from build123d import *

# Parameters (mm, degrees)
SKETCH1_W           = 48.698269881
SKETCH1_H           = 79.9
SKETCH1_W_2         = 13.312275424
SKETCH1_H_2         = 6.8
SKETCH1_W_3         = 7
SKETCH1_H_3         = 6.6
SKETCH1_W_4         = 10.999995004
SKETCH1_H_4         = 49.999979698
BOSS_EXTRUDE1_DEPTH = 6


with BuildPart() as part:
    # Sketch1 → Boss-Extrude1 (new body)
    with BuildSketch(Plane.XY):
        with Locations((-328.119749272, -326.315940756)):
            Rectangle(SKETCH1_W, SKETCH1_H)
        Polygon((-306.547681314, -310.331815037), (-306.727502074, -310.765940756), (-307.013555595, -311.138732962), (-307.386347801, -311.424786483), (-307.82047352, -311.604607243), (-308.286347801, -311.665940756), (-308.752222082, -311.604607243), (-309.186347801, -311.424786483), (-309.559140007, -311.138732962), (-309.845193528, -310.765940756), (-310.025014288, -310.331815037), (-310.086347801, -309.865940756), (-310.025014288, -309.400066475), (-309.845193528, -308.965940756), (-309.559140007, -308.59314855), (-309.186347801, -308.307095029), (-308.752222082, -308.127274269), (-308.286347801, -308.065940756), (-307.82047352, -308.127274269), (-307.386347801, -308.307095029), (-307.013555595, -308.59314855), (-306.727502074, -308.965940756), (-306.547681314, -309.400066475), (-306.486347801, -309.865940756), align=None, mode=Mode.SUBTRACT)
        with Locations((-314.125021924, -356.265940756)):
            Rectangle(SKETCH1_W_2, SKETCH1_H_2, mode=Mode.SUBTRACT)
        with Locations((-344.168884212, -356.165940756)):
            Rectangle(SKETCH1_W_3, SKETCH1_H_3, mode=Mode.SUBTRACT)
        with Locations((-314.125021924, -296.365940756)):
            Rectangle(SKETCH1_W_2, SKETCH1_H_2, mode=Mode.SUBTRACT)
        Polygon((-349.005509995, -349.753374061), (-349.195776334, -349.323723778), (-349.268357829, -348.859468921), (-349.218308171, -348.392247692), (-349.04903816, -347.953900444), (-348.77208327, -347.574299819), (-348.406317517, -347.279314973), (-347.976667234, -347.089048634), (-347.512412377, -347.016467139), (-347.045191148, -347.066516797), (-346.6068439, -347.235786808), (-346.227243275, -347.512741698), (-345.932258429, -347.878507451), (-345.74199209, -348.308157734), (-345.669410595, -348.772412591), (-345.719460253, -349.23963382), (-345.888730263, -349.677981068), (-346.165685154, -350.057581692), (-346.531450907, -350.352566539), (-346.96110119, -350.542832878), (-347.425356047, -350.615414373), (-347.892577276, -350.565364715), (-348.330924524, -350.396094704), (-348.710525148, -350.119139814), align=None, mode=Mode.SUBTRACT)
        Polygon((-307.013555595, -341.49314855), (-306.727502074, -341.865940756), (-306.547681314, -342.300066475), (-306.486347801, -342.765940756), (-306.547681314, -343.231815037), (-306.727502074, -343.665940756), (-307.013555595, -344.038732962), (-307.386347801, -344.324786483), (-307.82047352, -344.504607243), (-308.286347801, -344.565940756), (-308.752222082, -344.504607243), (-309.186347801, -344.324786483), (-309.559140007, -344.038732962), (-309.845193528, -343.665940756), (-310.025014288, -343.231815037), (-310.086347801, -342.765940756), (-310.025014288, -342.300066475), (-309.845193528, -341.865940756), (-309.559140007, -341.49314855), (-309.186347801, -341.207095029), (-308.752222082, -341.027274269), (-308.286347801, -340.965940756), (-307.82047352, -341.027274269), (-307.386347801, -341.207095029), align=None, mode=Mode.SUBTRACT)
        Polygon((-347.042471777, -302.06717764), (-346.604388229, -302.237128957), (-346.225218653, -302.51467369), (-345.93080283, -302.880897622), (-345.741204711, -303.310843199), (-345.669345095, -303.77521034), (-345.720121096, -304.242353191), (-345.890072413, -304.680436739), (-346.167617146, -305.059606315), (-346.533841078, -305.354022138), (-346.963786655, -305.543620257), (-347.428153795, -305.615479873), (-347.895296647, -305.564703872), (-348.333380195, -305.394752555), (-348.712549771, -305.117207822), (-349.006965594, -304.75098389), (-349.196563713, -304.321038313), (-349.268423329, -303.856671172), (-349.217647328, -303.389528321), (-349.047696011, -302.951444773), (-348.770151278, -302.572275197), (-348.403927346, -302.277859374), (-347.973981769, -302.088261255), (-347.509614628, -302.016401639), align=None, mode=Mode.SUBTRACT)
        with Locations((-344.168884212, -296.365940756)):
            Rectangle(SKETCH1_W_3, SKETCH1_H_2, mode=Mode.SUBTRACT)
        with Locations((-330.086347801, -326.315940756)):
            Rectangle(SKETCH1_W_4, SKETCH1_H_4, mode=Mode.SUBTRACT)
    extrude(amount=BOSS_EXTRUDE1_DEPTH)


solid = part.part
Could you check a few things on this model? Use its own coordinates, in mm. A direction names the side the tool comes from. Coordinates: 2 decimals unless noted, no trailing zeros. Loops run counter-clockwise (first coordinate to the right, second up) from the corner with the lowest first, then second, coordinate; pieces in that order, holes last.
1. Imagine slicing it at C-C (x = -333). Please give me the cut outline in (y, z), and give its area (3 significant figures).
2. I need wall thicknesses on L1, parallel to Y at x = -343, z = 1.8; L2, parallel to Y at x = -312.5, z = 0.6; L3, parallel to X at y = -332, z = 2.05. Which ranges of each line are inside material? Lowest first, please.
3. Imagine slicing it at D-D (z = 3.15). Give the number of separate pieces and of enclosed holes in the cut face, and give its area (3 significant figures).
4. Imagine slicing it at B-B (y = -330.5). Please give me the cut outline in (x, z).
5. Imagine slicing it at A-A (x = -314.5). Please give me the cut outline in (y, z).
6. For faces 3 (the face through (-344, -352.866, 3)), 4 (the face through (-323, -326, 6)), which set-ups out of +Z, -Z, +X, -X, +Y, -Y let a thin tool reach every point of the face, with its end or its side?
7. For P1, Ø6, axis at x = -337.5, y = -299, coming from the -Z side, with a flat end and sliding along its axis, tell me the tip position at first contact or that it passes through.
8. We'd pull the mould along Y, two halves only. Please class faces 1 (the face through (-335.586, -327, 3)), 2 (the face through (-323, -326, 0)): released by +Y, released by -Y, zero draft, split by the parting line, or undercut.
Computed values:
1. outline: (-366.27, 0) - (-351.32, 0) - (-351.32, 6) - (-366.27, 6) - close; (-301.32, 0) - (-286.37, 0) - (-286.37, 6) - (-301.32, 6) - close
1. area: 179 mm2
2. L1: y = -366.27 to -359.47, -352.87 to -299.77, -292.97 to -286.37
2. L2: y = -366.27 to -359.67, -352.87 to -299.77, -292.97 to -286.37
2. L3: x = -352.47 to -335.59, -324.59 to -303.77
3. separate pieces: 1
3. enclosed holes: 9
3. area: 3,030 mm2
4. outline: (-352.47, 0) - (-335.59, 0) - (-335.59, 6) - (-352.47, 6) - close; (-324.59, 0) - (-303.77, 0) - (-303.77, 6) - (-324.59, 6) - close
5. outline: (-366.27, 0) - (-359.67, 0) - (-359.67, 6) - (-366.27, 6) - close; (-352.87, 0) - (-299.77, 0) - (-299.77, 6) - (-352.87, 6) - close; (-292.97, 0) - (-286.37, 0) - (-286.37, 6) - (-292.97, 6) - close
6. face 3: +Z, -Z
6. face 4: +Z, +X, -X, +Y, -Y
7. P1: stops at z = 0
8. face 1: undercut
8. face 2: zero draft
